```python
from build123d import *

# Parameters (mm, degrees)
F0_R      = 11
F1_DEPTH  = 7
F2_R      = 9.5
F3_DEPTH  = 8
F4_R      = 4.25
F5_DEPTH  = 5.5
F6_R      = 3.25
F7_DEPTH  = 20.501
F8_R      = 2
F9_DEPTH  = 20.501
F12_R     = 2
F13_DEPTH = 6


# Not quite as in the source:
# - a feature names something its author has since deleted; it is built from what else it names


with BuildPart() as f1:
    # F0 (on Top) → F1 (new body)
    with BuildSketch(Plane.XY):
        Circle(F0_R)
    extrude(amount=F1_DEPTH)

    # F2 (on face) → F3 (join)
    with BuildSketch(Plane.XY.offset(7)):
        Circle(F2_R)
    extrude(amount=F3_DEPTH)

    # F4 (on face) → F5 (join)
    with BuildSketch(Plane.XY.offset(15)):
        Circle(F4_R)
    extrude(amount=F5_DEPTH)

    # F6 (on face) → F7 (cut, through all)
    with BuildSketch(Plane.XY.offset(20.5)):
        Circle(F6_R)
    extrude(amount=-F7_DEPTH, mode=Mode.SUBTRACT)

    # F8 (on face) → F9 (cut, through all)
    with BuildSketch(Plane(origin=(0, 0, 0), x_dir=(1, 0, 0), z_dir=(0, 0, -1))):
        with Locations((7, 0)):
            Circle(F8_R)
    extrude(amount=-F9_DEPTH, mode=Mode.SUBTRACT)

    # F12 (on line) → F13 (cut)
    with BuildSketch(Plane(origin=(-4.0535714286, -8.5917727317, 0), x_dir=(-0.9043971297, 0.4266917293, 0), z_dir=(0.4266917293, 0.9043971297, 0))):
        with Locations((0, 11)):
            Circle(F12_R)
    extrude(amount=F13_DEPTH, mode=Mode.SUBTRACT)


solid = f1.part
```
CAD build for the part. Positions are in the model's coordinates, mm. A direction names the side the tool comes from. Round coordinates to 2 decimals unless told otherwise and drop trailing zeros. Write each loop counter-clockwise with the first axis right and the second up, starting at its lowest first coordinate (ties: lowest second). Pieces come first, ordered by that corner, then holes. Notation, with made-up numbers: (12, 61.5) -> (24, 61.5) arc R25 ccw to (24, 97.5) -> close; hole circle Ø7 at (53, -8.75). An arc over 180 degrees is marked (long way). Answer in a Markdown table with one row per item. Add a question column.
Item 1: Saw through at D-D, the plane x = 0. Count the separate pieces of the cut face and the enclosed holes in it, then the cut area to 3 significant figures.
Item 2: Saw through at A-A, the plane y = 0. Write the cut outline in (x, z), then the cut area to 4 significant figures.
Item 3: Saw through at B-B, the plane x = 5.75. Write the cut outline in (y, z).
Item 4: Drill centre lines: line 1 (Y direction, x = 0, z = 10.25); line 2 (Z direction, x = -7.5, y = 1.75); line 3 (Y direction, x = 0, z = 14.75). Where is each one in solid material? Low to high. Write a range as from..to.
Item 5: Drop flat-ended pins along their axis: pin 1 Ø6 at (x, y) = (0, 0) entering from +Z; pin 2 Ø4 at (x, z) = (3, 9.5) entering from -Y; pin 3 Ø3 at (y, z) = (3, 15.5) entering from +X; pin 4 Ø1.5 at (x, z) = (-4, 5) entering from +Y. Give the stop position or say it passes through.
Item 6: Which spindle directions (+Z, -Z, +X, -X, +Y, -Y) get a long thin tool onto all of the face, cutting with end or side? Do faces 5 (the face through (4.38, -8.43, 10.94)), 6 (the face through (-2.579, -1.978, 10.394)). Say none if no direction does.
Item 7: Mould opens along Z. For faces 1 (the face through (-1.468, -3.177, 11.028)), 2 (the face through (2.285, 3.584, 17.712)), 3 (the face through (-10, 0, 7)), 4 (the face through (-3, -2, 0)) say: pulls with the +Z half, pulls with the -Z half, needs draft (parallel to the pull), parting line crosses it, or undercut.
Item 8: Saw through at C-C, the plane z = 9.5. Write the cut outline in (x, y).
Findings below:
| question | item | result |
|---|---|---|
| 1 | separate pieces | 2 |
| 1 | enclosed holes | 1 |
| 1 | area | 218 mm^2 |
| 2 | outline | (-11, 0) -> (-3.25, 0) -> (-3.25, 20.5) -> (-4.25, 20.5) -> (-4.25, 15) -> (-9.5, 15) -> (-9.5, 7) -> (-11, 7) -> close; (3.25, 0) -> (5, 0) -> (5, 15) -> (4.25, 15) -> (4.25, 20.5) -> (3.25, 20.5) -> close; (9, 0) -> (11, 0) -> (11, 7) -> (9.5, 7) -> (9.5, 15) -> (9, 15) -> close |
| 2 | area | 159.5 mm^2 |
| 3 | outline | (-9.38, 0) -> (-1.56, 0) -> (-1.56, 15) -> (-7.56, 15) -> (-7.56, 7) -> (-9.38, 7) -> close; (1.56, 0) -> (9.38, 0) -> (9.38, 7) -> (7.56, 7) -> (7.56, 15) -> (1.56, 15) -> close |
| 4 | line 1 | y = -9.5..-4.35, -3.87..-3.25, 3.25..9.5 |
| 4 | line 2 | z = 0..15 |
| 4 | line 3 | y = -9.5..-3.25, 3.25..9.5 |
| 5 | pin 1 | passes through |
| 5 | pin 2 | stops at y = -9.45 |
| 5 | pin 3 | stops at x = 9.37 |
| 5 | pin 4 | stops at y = 10.51 |
| 6 | face 5 | +Z |
| 6 | face 6 | +Z, -Z |
| 7 | face 1 | undercut |
| 7 | face 2 | needs draft |
| 7 | face 3 | pulls with the +Z half |
| 7 | face 4 | pulls with the -Z half |
| 8 | outline | (-5.21, -7.94) -> (-2.69, -2.6) -> (-0.3, -3.73) -> (-2.82, -9.07) arc R9.5 ccw (long way) to start; hole circle Ø6.5 at (0, 0); hole circle Ø4 at (7, 0) |
